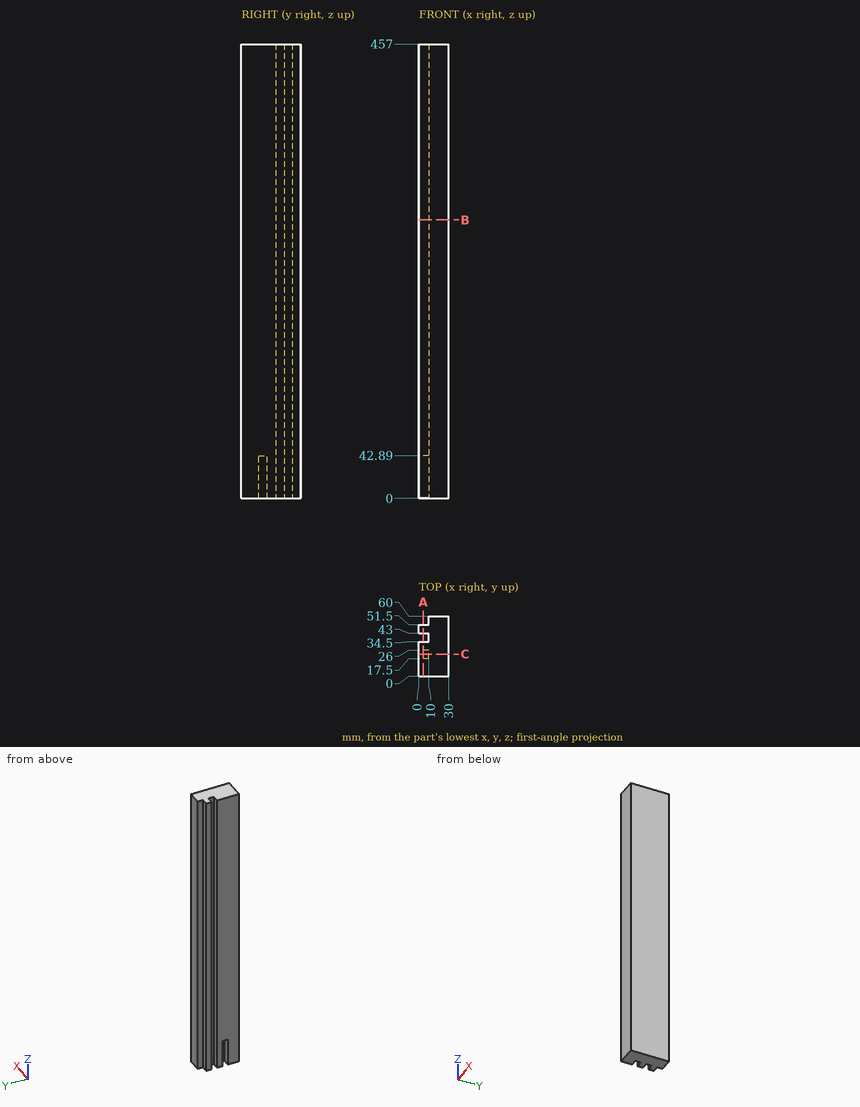
Here's the drawing with two shaded views (mm, measured from the low corner). I have some questions. Give positions to 0.01 mm unless a question says otherwise; leave off trailing zeros. Order: outer loops, then holes, each group sorted by start corner. A loop starts at its lowest first (then second) coordinate and runs counter-clockwise, first axis right, second up.
Q1. If I drill on line 1 along Y through (x, z) = (2, 39.5); line 2 along Y through (x, z) = (4, 70); line 3 along X through (y, z) = (38, 321), over which ranges is the centre line in solid material (lowest first)?
Q2. Suppose I cut it at A-A, the plane x = 4.5. Write out the boundary of the cut face in (y, z), and give its area (3 significant figures).
Q3. I'm going to push flat-ended pins straight in: P1, Ø2.5, axis at y = 22.5, z = 21, coming from the -X side; P2, Ø3, axis at x = 7.5, z = 19.5, coming from the +Y side. Where does each tip first touch, or does it pass through?
Q4. Suppose I cut it at B-B, the plane z = 280. Write out the boundary of the cut face in (x, y).
Q5. Suppose I cut it at C-C, the plane y = 22. Write out the boundary of the cut face in (x, z), and give its area (3 significant figures).
Solution:
1. line 1: y = 0 to 17.5, 26 to 34.5, 43 to 51.5
1. line 2: y = 0 to 34.5, 43 to 51.5
1. line 3: x = 10 to 30
2. outline: (0, 0) - (17.5, 0) - (17.5, 42.89) - (26, 42.89) - (26, 0) - (34.5, 0) - (34.5, 457) - (0, 457) - close; (43, 0) - (51.5, 0) - (51.5, 457) - (43, 457) - close
2. area: 19,300 mm2
3. P1: stops at x = 10
3. P2: stops at y = 51.5
4. outline: (0, 0) - (30, 0) - (30, 60) - (10, 60) - (10, 51.5) - (0, 51.5) - (0, 43) - (10, 43) - (10, 34.5) - (0, 34.5) - close
5. outline: (0, 42.89) - (10, 42.89) - (10, 0) - (30, 0) - (30, 457) - (0, 457) - close
5. area: 13,300 mm2
